For this review, take the finished solid that the model builds, in its own axes (mm). Round coordinates to 2 decimals unless told otherwise and drop trailing zeros. Loops run counter-clockwise (first coordinate to the right, second up) from the corner with the lowest first, then second, coordinate; pieces in that order, holes last. Notation, with made-up numbers: (60.25, 71.25) -> (109.25, 71.25) arc R26 ccw to (109.25, 86.25) -> close; hole circle Ø4 at (42.5, 89). An arc over 180 degrees is marked (long way). Write each question's results on one line, items separated by ' | '.
```python
from build123d import *

# Parameters (mm, degrees)
F0_W     = 103.632
F0_H     = 27.94
F1_DEPTH = 107.188
F2_R     = 26.162
F3_DEPTH = 27.941
F4_R     = 2.794
F5_DEPTH = 27.941
F6_R     = 1
F7_R     = 2


with BuildPart() as f1:
    # F0 (on Top) → F1 (new body)
    with BuildSketch(Plane.XY):
        Rectangle(F0_W, F0_H)
    extrude(amount=F1_DEPTH)

    # F2 (on face) → F3 (cut, through all)
    with BuildSketch(Plane.XZ.offset(13.97)):
        with Locations((0, 53.848)):
            Circle(F2_R)
    extrude(amount=-F3_DEPTH, mode=Mode.SUBTRACT)

    # F4 (on face) → F5 (cut, through all)
    with BuildSketch(Plane.XZ.offset(13.97)):
        with Locations((-39.243, 11.938)):
            Circle(F4_R)
        with Locations((39.243, 11.938)):
            Circle(F4_R)
    extrude(amount=-F5_DEPTH, mode=Mode.SUBTRACT)

    # F6
    f6_edges = [f1.edges().sort_by_distance(p)[0] for p in [
        (-26.162, -13.97, 53.848),
        (26.162, 0, 53.848),
        (-26.162, 13.97, 53.848),
    ]]
    fillet(f6_edges, radius=F6_R)

    # F7
    f7_edges = [f1.edges().sort_by_distance(p)[0] for p in [
        (51.816, 0, 107.188),
        (-51.816, 0, 107.188),
    ]]
    fillet(f7_edges, radius=F7_R)


solid = f1.part
```
1. Consider section A-A (x = 0). State the section outline as (y, z) points, plus the area to 3 significant figures.
Values found:
outline: (-13.97, 0) -> (13.97, 0) -> (13.97, 26.69) arc R1 ccw to (12.97, 27.69) -> (-12.97, 27.69) arc R1 ccw to (-13.97, 26.69) -> close; (-13.97, 81.01) arc R1 ccw to (-12.97, 80.01) -> (12.97, 80.01) arc R1 ccw to (13.97, 81.01) -> (13.97, 107.19) -> (-13.97, 107.19) -> close | area: 1,530 mm2
2. Consider section B-B (y = -0.5). State the section outline as (x, z) points, plus the area to 3 significant figures.
Values found:
outline: (-51.82, 0) -> (51.82, 0) -> (51.82, 105.19) arc R2 ccw to (49.82, 107.19) -> (-49.82, 107.19) arc R2 ccw to (-51.82, 105.19) -> close; hole circle Ø5.59 at (-39.24, 11.94); hole circle Ø52.32 at (0, 53.85); hole circle Ø5.59 at (39.24, 11.94) | area: 8,910 mm2
3. For pin 1 (5 mm diameter, centred on x = -39.243, z = 11.938, fed in from +Y), flat-tipped, find the tip position at first contact; note if it passes through.
Values found:
pin 1: passes through
4. Draft analysis for pull direction X (two halves, no side actions). For faces 1 (the face through (-12, -13.97, 29)), 2 (the face through (51.816, 0, 52)), 3 (the face through (40.53, -0.2, 9.46)), 4 (the face through (-3.406, -0.182, 79.787)), state which applies: released by +X, released by -X, zero draft, split by the parting line, or undercut.
Values found:
face 1: zero draft | face 2: released by +X | face 3: undercut | face 4: undercut
5. To check wall thickness, follow probe 1 along Z at (x, y) = (0, 0); probe 2 along X at (y, z) = (5, 48); probe 3 along X at (y, z) = (-8.5, 68). State the ranges of each line that lie inside material, in increasing order.
Values found:
probe 1: z = 0 to 27.69, 80.01 to 107.19 | probe 2: x = -51.82 to -25.5, 25.5 to 51.82 | probe 3: x = -51.82 to -22, 22 to 51.82
